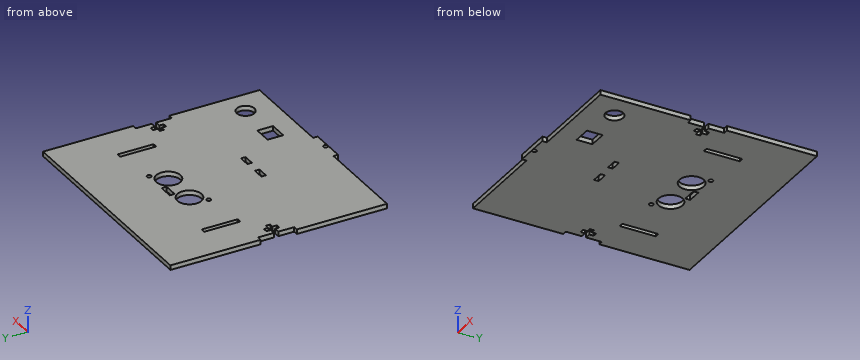
```python
from build123d import *

# Parameters (mm, degrees)
SKETCH1_R           = 1.5
BOSS_EXTRUDE1_DEPTH = 3.18
SKETCH2_R           = 6.1
SKETCH2_W           = 12.570473208
SKETCH2_H           = 10.91819785
CUT_EXTRUDE1_DEPTH  = 20
SKETCH4_R           = 8.384981778
SKETCH4_R_2         = 8.410411153
SKETCH4_W           = 9.999333355
SKETCH4_H           = 3.400001112
CUT_EXTRUDE2_DEPTH  = 10
SKETCH5_W           = 3.18
SKETCH5_H           = 25
SKETCH5_W_2         = 7.85
SKETCH5_H_2         = 3.18
CUT_EXTRUDE3_DEPTH  = 10
SKETCH8_R           = 1.5
CUT_EXTRUDE4_DEPTH  = 10


with BuildPart() as part:
    # Sketch1 → Boss-Extrude1 (new body)
    with BuildSketch(Plane.XY):
        Polygon((-78.18, 75), (78.18, 75), (78.18, 12.5), (75, 12.5), (75, 1.5), (71, 1.5), (71, 4.5), (68, 4.5), (68, 1.5), (65.18, 1.5), (65.18, -1.5), (68, -1.5), (68, -4.5), (71, -4.5), (71, -1.5), (75, -1.5), (75, -12.5), (78.18, -12.5), (78.18, -75), (12.5, -75), (12.5, -78.18), (-12.5, -78.18), (-12.5, -75), (-78.18, -75), (-78.18, -12.5), (-75, -12.5), (-75, -1.5), (-71, -1.5), (-71, -4.5), (-68, -4.5), (-68, -1.5), (-65.18, -1.5), (-65.18, 1.5), (-68, 1.5), (-68, 4.5), (-71, 4.5), (-71, 1.5), (-75, 1.5), (-75, 12.5), (-78.18, 12.5), align=None)
        with Locations(Location((0, -76.59, 0), (0, 0, 180))):
            Circle(SKETCH1_R, mode=Mode.SUBTRACT)
    extrude(amount=BOSS_EXTRUDE1_DEPTH)

    # Sketch2 → Cut-Extrude1 (cut)
    with BuildSketch(Plane.XY.offset(3.18)):
        with Locations((60.647779645, -55.45)):
            Circle(SKETCH2_R)
        with Locations((30.347779645, -55.45)):
            Rectangle(SKETCH2_W, SKETCH2_H)
    extrude(amount=-CUT_EXTRUDE1_DEPTH, mode=Mode.SUBTRACT)

    # Sketch4 → Cut-Extrude2 (cut)
    with BuildSketch(Plane.XY.offset(3.18)):
        with Locations((-12.93, 25)):
            Circle(SKETCH4_R)
        with Locations((12.93, 25)):
            Circle(SKETCH4_R_2)
        with Locations((0.003828225, 32.45)):
            Rectangle(SKETCH4_W, SKETCH4_H)
    extrude(amount=-CUT_EXTRUDE2_DEPTH, mode=Mode.SUBTRACT)

    # Sketch5 → Cut-Extrude3 (cut)
    with BuildSketch(Plane(origin=(0, 0, 0), x_dir=(-1, 0, 0), z_dir=(0, 0, -1))):
        with Locations((51.59, 25)):
            Rectangle(SKETCH5_W, SKETCH5_H)
        with Locations((-8.575, -26.59)):
            Rectangle(SKETCH5_W_2, SKETCH5_H_2)
        with Locations((8.575, -26.59)):
            Rectangle(SKETCH5_W_2, SKETCH5_H_2)
        with Locations((-51.59, 25)):
            Rectangle(SKETCH5_W, SKETCH5_H)
    extrude(amount=-CUT_EXTRUDE3_DEPTH, mode=Mode.SUBTRACT)

    # Sketch8 → Cut-Extrude4 (cut)
    with BuildSketch(Plane(origin=(0, 0, 0), x_dir=(-1, 0, 0), z_dir=(0, 0, -1))):
        with Locations((21.1, 16.25)):
            Circle(SKETCH8_R)
        with Locations((-21.1, 33.75)):
            Circle(SKETCH8_R)
    extrude(amount=-CUT_EXTRUDE4_DEPTH, mode=Mode.SUBTRACT)


solid = part.part
```
The model under review builds one solid part; all positions refer to its coordinate system, in mm. Coordinates: 2 decimals unless noted, no trailing zeros. Loops run counter-clockwise (first coordinate to the right, second up) from the corner with the lowest first, then second, coordinate; pieces in that order, holes last. Notation, with made-up numbers: (25, 62.25) -> (74, 62.25) arc R34 ccw to (74, 101.25) -> close; hole circle Ø8 at (37, -3.5). An arc over 180 degrees is marked (long way). Answer as CSV lines item,"result".
Item 1: Take a section at C-C, the plane z = 1.4. Count the separate pieces of the cut face and the enclosed holes in it, and give its area (3 significant figures).
Results below:
separate pieces,"1"
enclosed holes,"12"
area,"22,300 mm2"
Item 2: For L1, parallel to X at y = -28, z = 2; L2, parallel to X at y = -2.5, z = 1.8; L3, parallel to Y at x = -53, z = 0.8, list the stretches that pass through material, from the lowest coordinate up.
Results below:
L1,"x = -78.18 to -12.5, -4.65 to 4.65, 12.5 to 78.18"
L2,"x = -75 to -71, -68 to 68, 71 to 75"
L3,"y = -75 to 12.5, 37.5 to 75"
Item 3: Take a section at B-B, the plane y = -55.45. State the section outline as (x, z) points.
Results below:
outline,"(-78.18, 0) -> (24.06, 0) -> (24.06, 3.18) -> (-78.18, 3.18) -> close; (36.63, 0) -> (54.55, 0) -> (54.55, 3.18) -> (36.63, 3.18) -> close; (66.75, 0) -> (78.18, 0) -> (78.18, 3.18) -> (66.75, 3.18) -> close"
Item 4: Take a section at A-A, the plane x = 27. State the section outline as (y, z) points, and give its area (3 significant figures).
Results below:
outline,"(-75, 0) -> (-60.91, 0) -> (-60.91, 3.18) -> (-75, 3.18) -> close; (-49.99, 0) -> (75, 0) -> (75, 3.18) -> (-49.99, 3.18) -> close"
area,"442 mm2"
Item 5: Insertion check: pin 1 (1.6 mm diameter, centred on x = -52, z = 2, fed in from -Y); pin 2 (0.9 mm diameter, centred on y = -2.5, z = 1.5, fed in from +X). Each pin has a flat end and moves straight along its axis. Give the tip position at first contact, or say it passes through.
Results below:
pin 1,"stops at y = -75"
pin 2,"stops at x = 75"
Item 6: Take a section at D-D, the plane x = -48. State the section outline as (y, z) points, and give its area (3 significant figures).
Results below:
outline,"(-75, 0) -> (75, 0) -> (75, 3.18) -> (-75, 3.18) -> close"
area,"477 mm2"
